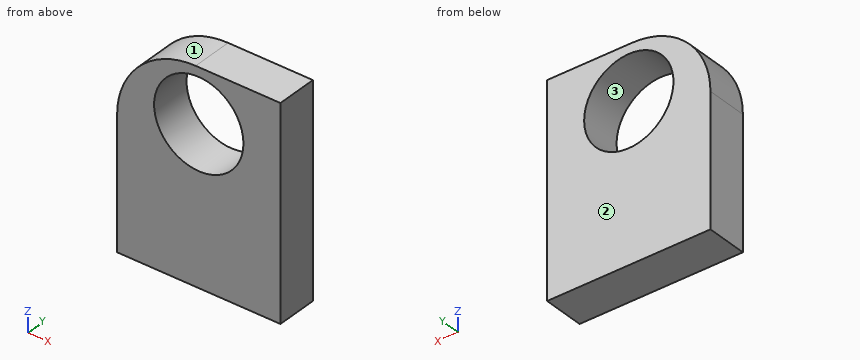
from build123d import *

# Parameters (mm, degrees)
F0_W     = 100.692854
F0_H     = 128.995716
F1_DEPTH = 25.4
F2_R     = 27.534887
F3_DEPTH = 170.942
F4_R     = 48.443609


with BuildPart() as f1:
    # F0 (on Front) → F1 (new body)
    with BuildSketch(Plane.XZ):
        Rectangle(F0_W, F0_H)
    extrude(amount=F1_DEPTH)

    # F2 (on Front) → F3 (cut)
    with BuildSketch(Plane.XZ):
        with Locations((0, 31.296428)):
            Circle(F2_R)
    extrude(amount=F3_DEPTH, mode=Mode.SUBTRACT)

    # F4
    f4_edges = [f1.edges().sort_by_distance(p)[0] for p in [
        (-50.346427, -12.7, 64.497858),
    ]]
    fillet(f4_edges, radius=F4_R)


solid = f1.part
Work out the finished part from the listing and answer in its coordinate system (mm). Face numbers are marked on the shaded views. Coordinates: 2 decimals unless noted, no trailing zeros. Order: outer loops, then holes, each group sorted by start corner. A loop starts at its lowest first (then second) coordinate and runs counter-clockwise, first axis right, second up. Notation, with made-up numbers: (77, -15.5) - (106, -15.5) arc R27 cw to (106, 2.5) - close; hole circle Ø3 at (69, -29.5). An arc over 180 degrees is marked (long way). Put each result on its own line as item: value. Start each with the question number.
1) Find the intervals of material crossed by line 1 (Z direction, x = 0, y = -19.5); line 2 (Z direction, x = -14.5, y = -18.5); line 3 (X direction, y = -4, z = 36), in increasing order. Write a range as from..to.
2) Find section D-D (x = -30). Give the vertices of the cut face in (y, z), plus the area to 3 significant figures.
3) A flat-ended cylindrical pin translates along its axis: pin 1 (4 mm diameter, centred on x = -5, y = -17.5, fed in from +Z). Find the tip coordinate at first contact, or state that the pin passes through.
4) Find section C-C (y = -4.75). Give the vertices of the cut face in (x, z), plus the area to 3 significant figures.
5) For a pull along X with two mould halves and no side action, classify the marked faces 1, 2 and 3 as released by +X, released by -X, zero draft, split by the parting line, or undercut.
6) Find section B-B (z = 40). Give the vertices of the cut face in (x, y).
7) Find section A-A (x = 0). Give the vertices of the cut face in (y, z), plus the area to 3 significant figures.
Results list:
1. line 1: z = -64.5..3.76, 58.83..64.5
1. line 2: z = -64.5..7.89, 54.7..62.83
1. line 3: x = -46.05..-27.13, 27.13..50.35
2. outline: (-25.4, -64.5) - (0, -64.5) - (0, 55.52) - (-25.4, 55.52) - close
2. area: 3,050 mm^2
3. pin 1: stops at z = 64.49
4. outline: (-50.35, -64.5) - (50.35, -64.5) - (50.35, 64.5) - (-1.9, 64.5) arc R48.44 ccw to (-50.35, 16.05) - close; hole circle Ø55.07 at (0, 31.3)
4. area: 10,100 mm^2
5. face 1: released by -X
5. face 2: zero draft
5. face 3: undercut
6. outline: (-44.01, -25.4) - (-26.12, -25.4) - (-26.12, 0) - (-44.01, 0) - close; (26.12, -25.4) - (50.35, -25.4) - (50.35, 0) - (26.12, 0) - close
7. outline: (-25.4, -64.5) - (0, -64.5) - (0, 3.76) - (-25.4, 3.76) - close; (-25.4, 58.83) - (0, 58.83) - (0, 64.5) - (-25.4, 64.5) - close
7. area: 1,880 mm^2
